```python
from build123d import *

# Parameters (mm, degrees)
F1_DEPTH = 100
F2_R     = 1.99999


# Not quite as in the source:
# - a fillet or chamfer is up to 0.001 mm smaller than in the source, because OpenCascade refuses the exact size


with BuildPart() as f1:
    # F0 (on Right) → F1 (new body)
    with BuildSketch(Plane.YZ):
        Polygon((33, -23), (35, -23), (35, 0), (0, 0), (0, -95), (28, -95), (28, -80), (15.1442478063, -64.6791111376), (15.1442478063, -51.1349920747), (29.9283628291, -33.5159698829), (29.9283628291, -23.5159698829), (27.9283628291, -23.5159698829), (27.9283628291, -32.7880294144), (13.1442478063, -50.4070516062), (13.1442478063, -65.4070516062), (26, -80.7279404685), (26, -93), (2, -93), (2, -2), (33, -2), align=None)
    extrude(amount=F1_DEPTH)

    # F2 (radius 2 in the source; OpenCascade refuses exactly that, so slightly less here)
    f2_edges = [f1.edges().sort_by_distance(p)[0] for p in [
        (50, 35, 0),
        (50, 0, 0),
        (50, 33, -2),
        (50, 2, -2),
        (50, 0, -95),
        (50, 28, -95),
        (50, 28, -80),
        (50, 2, -93),
        (50, 26, -93),
        (50, 26, -80.72794),
        (50, 27.928363, -32.788029),
        (50, 15.144248, -64.679111),
        (50, 29.928363, -33.51597),
        (50, 29.928363, -23.51597),
        (50, 13.144248, -50.407052),
        (50, 13.144248, -65.407052),
    ]]
    fillet(f2_edges, radius=F2_R)


solid = f1.part
```
Check sheet for the modelled part. Datum: model origin and axes. Units: mm. A direction names the side the tool comes from. Give positions to 0.01 mm unless a question says otherwise; leave off trailing zeros. Loops run counter-clockwise (first coordinate to the right, second up) from the corner with the lowest first, then second, coordinate; pieces in that order, holes last. Notation, with made-up numbers: (55, 71.5) - (75, 71.5) arc R17 ccw to (75, 100.5) - close; hole circle Ø5 at (-21, 22.5). An arc over 180 degrees is marked (long way). One line per question, with ' | ' between items. Start each with the question number.
1. Draft check along Y on faces 5 (the flat face through (49, 13.144, -58)), 6 (the flat face through (49, 0, -47)), 7 (the flat face through (49, 29.928, -29)). Enter one of: released by +Y, released by -Y, zero draft, split by the parting line, or undercut.
2. Gauge pin test, flat ends, axial feed: pin 1 Ø2 at (x, z) = (73.5, -28) entering from +Y; pin 2 Ø12 at (x, z) = (47.5, -81.5) entering from +Y; pin 3 Ø5 at (y, z) = (19.5, -66.5) entering from +X; pin 4 Ø1.5 at (x, z) = (88.5, -78.5) entering from +Y. Record the tip position at first contact, or that the pin passes through.
3. Cross-section at B-B, the plane y = 9.5. Enter the section's corners in (x, z).
4. Cross-section at A-A, the plane z = -53. Enter the section's corners in (x, y), plus the area to 3 significant figures.
5. Cross-section at C-C, the plane y = 19. Enter the section's corners in (x, z), plus the area to 3 significant figures.
6. Material ranges on line 1 along Y through (x, z) = (51.5, -18); line 2 along Z through (x, y) = (82, 9); line 3 along Y through (x, z) = (48, -31), recorded low to high. Write a range as [from, to].
7. Set-up check for faces 1 (the flat face through (49, 2, -48)), 2 (the flat face through (49, 28, -87)), 3 (the flat face through (49, 33, -13)), 4 (the flat face through (49.3, 21.656, -72.439)): record each of +Z, -Z, +X, -X, +Y, -Y from which the full face is reachable in a straight line by a thin tool's end or side.
Check result:
1) face 5: undercut | face 6: released by -Y | face 7: released by +Y
2) pin 1: stops at y = 29.93 | pin 2: stops at y = 28 | pin 3: stops at x = 100 | pin 4: stops at y = 27.37
3) outline: (0, -95) - (100, -95) - (100, -93) - (0, -93) - close; (0, -2) - (100, -2) - (100, 0) - (0, 0) - close
4) outline: (0, 0) - (100, 0) - (100, 2) - (0, 2) - close; (0, 13.14) - (100, 13.14) - (100, 15.14) - (0, 15.14) - close | area: 400 mm2
5) outline: (0, -95) - (100, -95) - (100, -93) - (0, -93) - close; (0, -72.39) - (100, -72.39) - (100, -69.27) - (0, -69.27) - close; (0, -46.54) - (100, -46.54) - (100, -43.43) - (0, -43.43) - close; (0, -2) - (100, -2) - (100, 0) - (0, 0) - close | area: 1,020 mm2
6) line 1: y = [0, 2], [33, 35] | line 2: z = [-95, -93], [-2, 0] | line 3: y = [0, 2], [27.93, 29.93]
7) face 1: +X, -X | face 2: -Z, +X, -X, +Y | face 3: -Z, +X, -X | face 4: +X, -X, +Y
